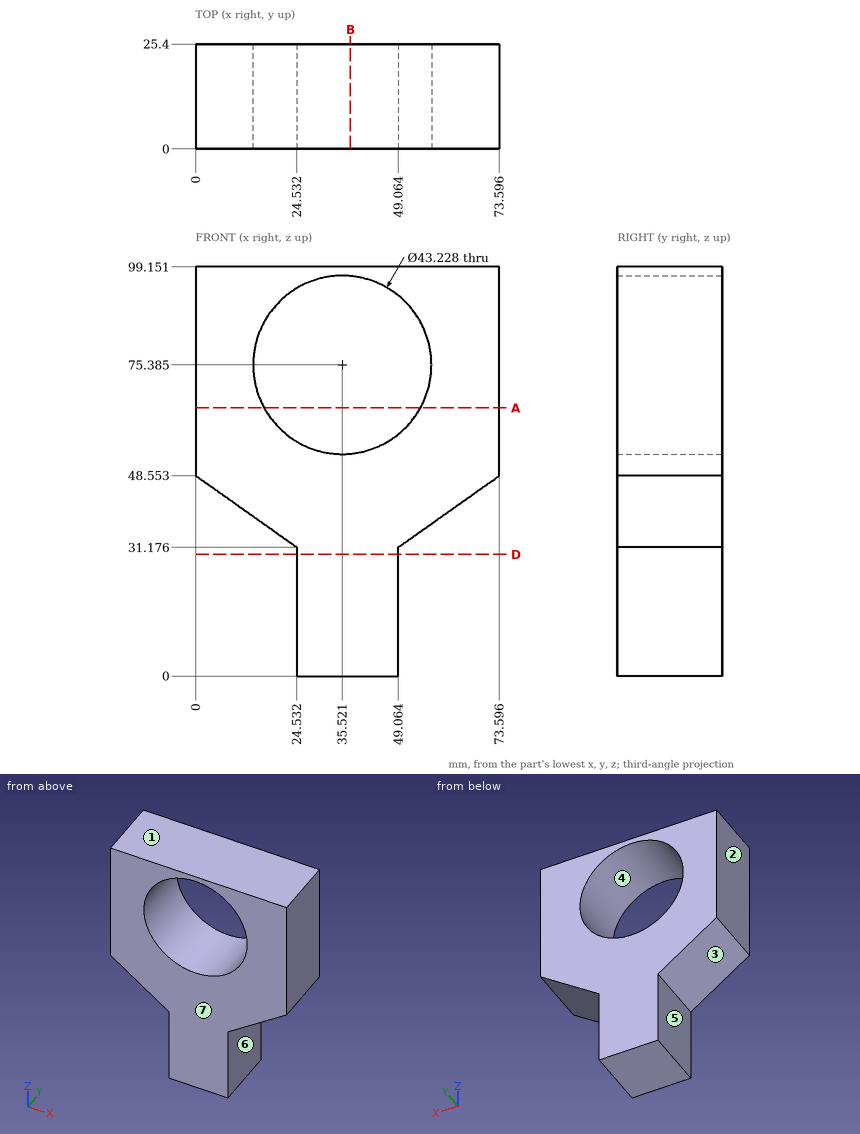
Input: dimensioned drawing with shaded views. Units: mm. Origin: part minimum x, y, z. A direction names the side the tool comes from. Coordinates: 2 decimals unless noted, no trailing zeros. Loops run counter-clockwise (first coordinate to the right, second up) from the corner with the lowest first, then second, coordinate; pieces in that order, holes last. Notation, with made-up numbers: (71.25, 5.25) - (111.25, 5.25) arc R16 cw to (111.25, 13.25) - close; hole circle Ø6 at (21.25, 89). An arc over 180 degrees is marked (long way). One line per question, with ' | ' between items. Start each with the question number.
(1) Cut plane B-B on x = 37.5. Output: boundary loops of the cut face in (y, z).
(2) Cut plane D-D on z = 29.5. Output: boundary loops of the cut face in (x, y) (1 decimal), and give its area (3 significant figures).
(3) Cut plane A-A on z = 65. Output: boundary loops of the cut face in (x, y) (1 decimal).
(4) Ray query, L1, parallel to X at y = 10.5, z = 75; L2, parallel to X at y = 18.5, z = 29.5 (1 decimal); L3, parallel to X at y = 10, z = 61.5 (1 decimal). Return the intervals inside material, ascending. Write a range as from..to.
(5) Reachability of the marked faces 5, 6 and 7 from +Z, -Z, +X, -X, +Y, -Y: full face, straight path, thin tool, end or side. Return the list, or none.
(6) First-contact query: pin 1 (3 mm diameter, centred on y = 8, z = 27.5, fed in from -X); pin 2 (3 mm diameter, centred on y = 7.5, z = 33.5, fed in from -X) (1 decimal); pin 3 (7.5 mm diameter, centred on y = 11.5, z = 10, fed in from +X). Flat tips, straight axial feed; report the tip coordinate or a pass-through.
(7) Draft query along Z for the marked faces 1, 2, 3 and 4. Return one class per face: +Z half, -Z half, draft (parallel to the pull), parting line (faces both ways), or undercut.
Here are the results:
1) outline: (0, 0) - (25.4, 0) - (25.4, 53.86) - (0, 53.86) - close; (0, 96.91) - (25.4, 96.91) - (25.4, 99.15) - (0, 99.15) - close
2) outline: (24.5, 0) - (49.1, 0) - (49.1, 25.4) - (24.5, 25.4) - close | area: 623 mm²
3) outline: (0, 0) - (16.6, 0) - (16.6, 25.4) - (0, 25.4) - close; (54.5, 0) - (73.6, 0) - (73.6, 25.4) - (54.5, 25.4) - close
4) L1: 0..13.91, 57.13..73.6 | L2: 24.5..49.1 | L3: 0..19, 52.1..73.6
5) face 5: -Z, -X, +Y, -Y | face 6: -Z, +X, +Y, -Y | face 7: +Z, -Z, +X, -X, -Y
6) pin 1: x = 24.53 | pin 2: x = 19.1 | pin 3: x = 49.06
7) face 1: +Z half | face 2: draft | face 3: -Z half | face 4: undercut
